Autodesk Fusion 360 part; units mm, degrees
sketch "Sketch1" plane through (0, 0, 0) normal (0, 0, 1) x (1, 0, 0)
  line L0 (0, 49.25) -> (40, 49.25)
  line L1 (40, 49.25) -> (40, 19.25)
  line L2 (40, 19.25) -> (60, 19.25)
  line L3 (60, 19.25) -> (60, 0)
  line L4 (0, -52) -> (30, -52)
  arc A0 (30, -52) -> (60, 0) centre (-0.0667, 0) ccw
  circle A1 centre (15.875, 39.25) radius 2.1
  circle A2 centre (45, 0) radius 1.6
  circle A3 centre (24.6, -44.1599) radius 2.1
  circle A4 centre (-45, 0) radius 1.6
  line L5 (-60, 14.25) -> (-60, 0)
  arc A5 (-60, 0) -> (-30, -52) centre (0.0667, 0) ccw
  line L6 (0, -52) -> (-30, -52)
  line L7 (0, 49.25) -> (-40, 49.25)
  circle A6 centre (0.0667, 0) radius 32.5
  line L8 (-40, 49.25) -> (-40, 19.25)
  line L9 (-40, 19.25) -> (-60, 19.25)
  line L10 (-60, 19.25) -> (-60, 14.25)
  circle A7 centre (-24.6, -44.1599) radius 2.1
  circle A8 centre (-15.875, 39.25) radius 2.1
  dimension "d1" = 49.25
  dimension "d2" = 40
  dimension "d3" = 30
  dimension "d4" = 20
  dimension "d5" = 52
  dimension "d6" = 30
  dimension "d12" = 4.2
  dimension "d13" = 45
  dimension "d14" = 3.2
  dimension "d17" = 4.2
  dimension "d20" = 65
  dimension "d23" = 30
  dimension "d24" = 4.2
  dimension "d25" = 4.2
extrude "Extrude4" add sketch "Sketch1" along normal blind 6.35
Geometry: final body of the model. Coordinates: model frame, mm. A direction names the side the tool comes from. Coordinates: 2 decimals unless noted, no trailing zeros. Order: outer loops, then holes, each group sorted by start corner. A loop starts at its lowest first (then second) coordinate and runs counter-clockwise, first axis right, second up. Notation, with made-up numbers: M 78,38 L 91,38 A30 ccw 91,70 Z; hole C 77,-34 d5. An arc over 180 degrees is marked long. Answer as CSV lines item,"result".
Q1. Section D-D on x = -45. Return the cut outline in (y, z).
Answers:
outline,"M -39.71,0 L -1.6,0 L -1.6,6.35 L -39.71,6.35 Z; M 1.6,0 L 19.25,0 L 19.25,6.35 L 1.6,6.35 Z"
Q2. Section A-A on y = 39.25. Return the cut outline in (x, z) (3 decimals).
Answers:
outline,"M -40,0 L -17.975,0 L -17.975,6.35 L -40,6.35 Z; M -13.775,0 L 13.775,0 L 13.775,6.35 L -13.775,6.35 Z; M 17.975,0 L 40,0 L 40,6.35 L 17.975,6.35 Z"
Q3. Line query: probe 1 along Y at (x, z) = (17, 0.75); probe 2 along Y at (x, z) = (-45, 3.25); probe 3 along X at (y, z) = (-16.5, 1.75). Output: solid intervals per line, ascending. Write a range as [from, to].
Answers:
probe 1,"y = [-52, -27.74], [27.74, 37.48], [41.02, 49.25]"
probe 2,"y = [-39.71, -1.6], [1.6, 19.25]"
probe 3,"x = [-57.69, -27.93], [28.07, 57.69]"
Q4. First-contact query: P1, Ø3, axis at y = 37, z = 3, coming from the -X side; P2, Ø3, axis at x = -48.5, z = 3.5, coming from the +Y side; P3, Ø3.5, axis at x = -15.875, y = 39.25, coming from the -Z side; P4, Ø1.5, axis at x = -40, z = 4, coming from the -Y side. Flat tips, straight axial feed; report the tip coordinate or a pass-through.
Answers:
P1,"stops at x = -40"
P2,"stops at y = 19.25"
P3,"passes through"
P4,"stops at y = -45.41"
Q5. Draft query along X for faces 4 (the cylindrical face through (-24.873, -46.242, 3.131)), 5 (the cylindrical face through (-46.18, -1.08, 3.13)), 6 (the flat face through (-40, 34, 3)), 7 (the flat face through (0, -52, 3)). Return one class per face: pulls with the +X half, pulls with the -X half, needs draft (parallel to the pull), parting line crosses it, or undercut.
Answers:
face 4,"undercut"
face 5,"undercut"
face 6,"pulls with the -X half"
face 7,"needs draft"
Q6. Section B-B on x = 24.6. Return the cut outline in (y, z).
Answers:
outline,"M -52,0 L -46.26,0 L -46.26,6.35 L -52,6.35 Z; M -42.06,0 L -21.32,0 L -21.32,6.35 L -42.06,6.35 Z; M 21.32,0 L 49.25,0 L 49.25,6.35 L 21.32,6.35 Z"
Q7. Section C-C on z = 4.5. Return the cut outline in (x, y) (3 decimals), and give its area (3 significant figures).
Answers:
outline,"M -60,0 A60.067 ccw -30,-52 L 30,-52 A60.067 ccw 60,0 L 60,19.25 L 40,19.25 L 40,49.25 L -40,49.25 L -40,19.25 L -60,19.25 Z; hole C -45,0 d3.2; hole C 0.067,0 d65; hole C -24.6,-44.16 d4.2; hole C -15.875,39.25 d4.2; hole C 15.875,39.25 d4.2; hole C 24.6,-44.16 d4.2; hole C 45,0 d3.2"
area,"6,650 mm^2"
Q8. Set-up query: faces 1 (the flat face through (60, 10, 3)), 2 (the flat face through (40, 34, 3)), 3 (the flat face through (-50, 19.25, 3)). Return all of +Z, -Z, +X, -X, +Y, -Y with unobstructed straight access to the full face (end or side cutting, diameter ignored); none if empty.
Answers:
face 1,"+Z, -Z, +X, +Y, -Y"
face 2,"+Z, -Z, +X, +Y"
face 3,"+Z, -Z, -X, +Y"
